from build123d import *

# Parameters (mm, degrees)
SKETCH_1_R          = 1.8
SKETCH_1_R_2        = 6.55
SKETCH_1_R_3        = 2.7
SKETCH_1_W          = 20.4
SKETCH_1_H          = 20.4
EXTRUDE_1_DEPTH     = 4
EXTRUDE_START       = 4
SKETCH_1_4_W        = 32
SKETCH_1_4_H        = 30
SKETCH_1_4_W_2      = 20.4
SKETCH_1_4_H_2      = 20.4
SKETCH_1_4_R        = 1.6
EXTRUDE_3_DEPTH     = 19.6
CUT_EXTRUDE_4_REACH = 103.812
SKETCH_8_R          = 2.2
SKETCH_9_R          = 5
SKETCH_9_R_2        = 2.7
EXTRUDE_4_DEPTH     = 7.5


with BuildPart() as part:
    # 草图1 → 凸台-拉伸1 (new body)
    with BuildSketch(Plane.XY):
        with BuildLine():
            ThreePointArc((-36, -25.5), (-31.606601718, -36.106601718), (-21, -40.5))
            Line((-21, -40.5), (21, -40.5))
            ThreePointArc((21, -40.5), (31.606601718, -36.106601718), (36, -25.5))
            Line((36, -25.5), (36, -14.520797289))
            ThreePointArc((36, -14.520797289), (38.5, -8.5), (36, -2.479202711))
            Line((36, -2.479202711), (36, 32.75))
            ThreePointArc((36, 32.75), (30.727922061, 45.477922061), (18, 50.75))
            Line((18, 50.75), (-18, 50.75))
            ThreePointArc((-18, 50.75), (-30.727922061, 45.477922061), (-36, 32.75))
            Line((-36, 32.75), (-36, -2.479202711))
            ThreePointArc((-36, -2.479202711), (-38.5, -8.5), (-36, -14.520797289))
            Line((-36, -14.520797289), (-36, -25.5))
        make_face()
        with Locations((15.5, -35)):
            Circle(SKETCH_1_R, mode=Mode.SUBTRACT)
        with Locations((0, -19.5)):
            Circle(SKETCH_1_R_2, mode=Mode.SUBTRACT)
        with Locations((15.5, -4)):
            Circle(SKETCH_1_R, mode=Mode.SUBTRACT)
        with Locations((-15.5, -35)):
            Circle(SKETCH_1_R, mode=Mode.SUBTRACT)
        with Locations((-15.5, -4)):
            Circle(SKETCH_1_R, mode=Mode.SUBTRACT)
        with Locations((-30, -8.5)):
            Circle(SKETCH_1_R_3, mode=Mode.SUBTRACT)
        with Locations((30, -8.5)):
            Circle(SKETCH_1_R_3, mode=Mode.SUBTRACT)
        with Locations((-29, 28.1)):
            Circle(SKETCH_1_R_3, mode=Mode.SUBTRACT)
        with Locations((29, 28.1)):
            Circle(SKETCH_1_R_3, mode=Mode.SUBTRACT)
        with Locations((0, 35.75)):
            Rectangle(SKETCH_1_W, SKETCH_1_H, mode=Mode.SUBTRACT)
    extrude(amount=EXTRUDE_1_DEPTH)

    # 草图1<4> → 凸台-拉伸3 (add)
    # profile 1 of 3: a face of its own
    with BuildSketch(Plane.XY.offset(EXTRUDE_START)):
        with Locations((0, 35.75)):
            Rectangle(SKETCH_1_4_W, SKETCH_1_4_H)
        with Locations((0, 35.75)):
            Rectangle(SKETCH_1_4_W_2, SKETCH_1_4_H_2, mode=Mode.SUBTRACT)
    # profile 2 of 3: a face of its own
    with BuildSketch(Plane.XY.offset(EXTRUDE_START)):
        with Locations((-13.2, 35.75)):
            Circle(SKETCH_1_4_R)
    # profile 3 of 3: a face of its own
    with BuildSketch(Plane.XY.offset(EXTRUDE_START)):
        with Locations((13.2, 35.75)):
            Circle(SKETCH_1_4_R)
    extrude(amount=EXTRUDE_3_DEPTH)

    # 草图8 → 切除-拉伸4 (cut, up to next)
    with BuildSketch(Plane(origin=(0, 50.75, 0), x_dir=(1, 0, 0), z_dir=(0, 1, 0)), mode=Mode.PRIVATE) as cut_extrude_4_sk1:
        with Locations(Location((0, -14, 0), (0, 0, 270))):
            Circle(SKETCH_8_R)
    cut_extrude_4_tool1 = extrude(cut_extrude_4_sk1.sketch, amount=-CUT_EXTRUDE_4_REACH, mode=Mode.PRIVATE) & part.part
    add(cut_extrude_4_tool1.solids().sort_by_distance((0, 50.75, 14))[0], mode=Mode.SUBTRACT)

    # 草图9 → 凸台-拉伸4 (add)
    # profile 1 of 4: a face of its own
    with BuildSketch(Plane.XY.offset(4)):
        with Locations((-29, 28.1)):
            Circle(SKETCH_9_R)
        with Locations((-29, 28.1)):
            Circle(SKETCH_9_R_2, mode=Mode.SUBTRACT)
    # profile 2 of 4: a face of its own
    with BuildSketch(Plane.XY.offset(4)):
        with Locations((-30, -8.5)):
            Circle(SKETCH_9_R)
        with Locations((-30, -8.5)):
            Circle(SKETCH_9_R_2, mode=Mode.SUBTRACT)
    # profile 3 of 4: a face of its own
    with BuildSketch(Plane.XY.offset(4)):
        with Locations(Location((30, -8.5, 0), (0, 0, 180))):
            Circle(SKETCH_9_R)
        with Locations(Location((30, -8.5, 0), (0, 0, 180))):
            Circle(SKETCH_9_R_2, mode=Mode.SUBTRACT)
    # profile 4 of 4: a face of its own
    with BuildSketch(Plane.XY.offset(4)):
        with Locations(Location((29, 28.1, 0), (0, 0, 180))):
            Circle(SKETCH_9_R)
        with Locations(Location((29, 28.1, 0), (0, 0, 180))):
            Circle(SKETCH_9_R_2, mode=Mode.SUBTRACT)
    extrude(amount=EXTRUDE_4_DEPTH)


solid = part.part
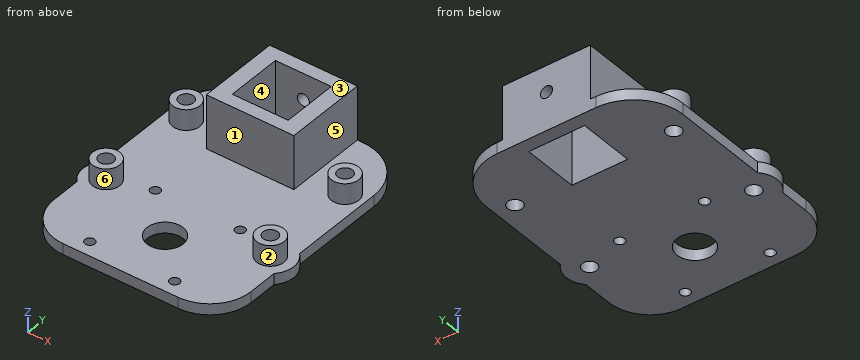
The model under review builds one solid part; all positions refer to its coordinate system, in mm. Face numbers are marked on the shaded views. A direction names the side the tool comes from. Coordinates: 2 decimals unless noted, no trailing zeros. Loops run counter-clockwise (first coordinate to the right, second up) from the corner with the lowest first, then second, coordinate; pieces in that order, holes last. Notation, with made-up numbers: (-24.75, -35.5) -> (8.25, -35.5) arc R9 cw to (8.25, -21.5) -> close; hole circle Ø5 at (-20, 87.25). An arc over 180 degrees is marked (long way). Use a Markdown table: item, result. Add a question column.
1. Add section C-C on x = 30. Write out the cut boundary in (y, z).
2. Add section B-B on z = 19.5. Write out the cut boundary in (x, y).
3. Add section D-D on y = -35. Write out the cut boundary in (x, z), plus the area to 3 significant figures.
4. Draft analysis for pull direction Y (two halves, no side actions). For the marked faces 1, 2 and 3, state which applies: pulls with the +Y half, pulls with the -Y half, needs draft (parallel to the pull), parting line crosses it, or undercut.
5. Machinability: for the marked faces 4, 5 and 6, which of the approach directions +Z, -Z, +X, -X, +Y, -Y give a long, thin tool a straight path to every point of the face, cutting with its end or side? Answer none if there is none.
6. Add section A-A on y = -19.5. Write out the cut boundary in (x, z), plus the area to 3 significant figures.
7. To check wall thickness, follow line 1 (Y direction, x = -15.5, z = 1.1); line 2 (Y direction, x = -3, z = 1); line 3 (Y direction, x = -7.5, z = 8.5). State the ranges of each line that lie inside material, in increasing order.
8. Clearance check with flat-ended pins moving along their axes: pin 1 Ø11 at (x, y) = (-27, 29.5) entering from +Z; pin 2 Ø3 at (y, z) = (-21.5, 1) entering from -X; pin 3 Ø6 at (y, z) = (-28.5, 4.5) entering from +X. State where each tip first meets the part, or that it passes through.
Returned:
| question | item | result |
|---|---|---|
| 1 | outline | (-37.5, 0) -> (-11.2, 0) -> (-11.2, 11.5) -> (-13.5, 11.5) -> (-13.5, 4) -> (-37.5, 4) -> close; (-5.8, 0) -> (25.59, 0) -> (25.59, 11.5) -> (23.2, 11.5) -> (23.2, 4) -> (-3.5, 4) -> (-3.5, 11.5) -> (-5.8, 11.5) -> close; (30.61, 0) -> (46.17, 0) -> (46.17, 4) -> (33, 4) -> (33, 11.5) -> (30.61, 11.5) -> close |
| 2 | outline | (-16, 20.75) -> (16, 20.75) -> (16, 50.75) -> (-16, 50.75) -> close; hole (-10.2, 25.55) -> (10.2, 25.55) -> (10.2, 45.95) -> (-10.2, 45.95) -> close |
| 3 | outline | (-32.61, 0) -> (-17.3, 0) -> (-17.3, 4) -> (-32.61, 4) -> close; (-13.7, 0) -> (13.7, 0) -> (13.7, 4) -> (-13.7, 4) -> close; (17.3, 0) -> (32.61, 0) -> (32.61, 4) -> (17.3, 4) -> close |
| 3 | area | 232 mm² |
| 4 | face 1 | pulls with the -Y half |
| 4 | face 2 | undercut |
| 4 | face 3 | needs draft |
| 5 | face 4 | +Z, -Z |
| 5 | face 5 | +Z, +Y, -Y |
| 5 | face 6 | +Z |
| 6 | outline | (-36, 0) -> (-6.55, 0) -> (-6.55, 4) -> (-36, 4) -> close; (6.55, 0) -> (36, 0) -> (36, 4) -> (6.55, 4) -> close |
| 6 | area | 236 mm² |
| 7 | line 1 | y = -40.5 to -36.8, -33.2 to -5.8, -2.2 to 50.75 |
| 7 | line 2 | y = -40.5 to -25.32, -13.68 to 25.55, 45.95 to 50.75 |
| 7 | line 3 | y = 20.75 to 25.55, 45.95 to 50.75 |
| 8 | pin 1 | stops at z = 11.5 |
| 8 | pin 2 | stops at x = -36 |
| 8 | pin 3 | stops at x = 36 |
